Part model, mm, in its own coordinate system. Face numbers are marked on the shaded views. A direction names the side the tool comes from. Coordinates: 2 decimals unless noted, no trailing zeros. Loops run counter-clockwise (first coordinate to the right, second up) from the corner with the lowest first, then second, coordinate; pieces in that order, holes last. Notation, with made-up numbers: M 30,2.5 L 84,2.5 A9 cw 84,9.5 Z; hole C 8,42.5 d6. An arc over 180 degrees is marked long. Use a Markdown table: item, result. Add a question column.
1) Pin check, flat tips, straight feed: pin 1 Ø9.5 at (x, z) = (22, 0) entering from -Y; pin 2 Ø1 at (y, z) = (1, 0.5) entering from +X; pin 3 Ø6 at (x, z) = (5, -7) entering from +Y. Stop position of each tip, or through.
2) Band-saw the part on A-A (y = 1.25). List the corners of the cut face in (x, z), plus the area to 3 significant figures.
3) Band-saw the part on C-C (z = 2). List the corners of the cut face in (x, y), plus the area to 3 significant figures.
4) Pull direction X, two halves, no side cores. Call the marked faces 3, 4 and 5: released by +X, released by -X, zero draft, split by the parting line, or undercut.
5) Tool access for the marked faces 1 and 2: list every direction of +Z, -Z, +X, -X, +Y, -Y with a clear straight run to the whole face (end or side of a thin tool).
6) Wall check: probe 1 along X at (y, z) = (13.5, -7); probe 2 along Y at (x, z) = (29.5, 1.5); probe 3 along Y at (x, z) = (13.5, 10). Give the ranges that are in metal, low to high. Write a range as from..to.
7) Band-saw the part on B-B (x = 0). List the corners of the cut face in (y, z), plus the area to 3 significant figures.
from build123d import *

# Parameters (mm, degrees)
SKETCH_1_W          = 64
SKETCH_1_H          = 36
EXTRUDE_1_DEPTH     = 15.3
SKETCH_2_W          = 44
SKETCH_2_H          = 25
CUT_EXTRUDE_1_DEPTH = 2
SKETCH_3_W          = 16
SKETCH_3_H          = 6
CUT_EXTRUDE_2_DEPTH = 2


with BuildPart() as part:
    # 草图1 → 凸台-拉伸1 (new body)
    with BuildSketch(Plane(origin=(0, 0, 0), x_dir=(1, 0, 0), z_dir=(0, 1, 0))):
        Rectangle(SKETCH_1_W, SKETCH_1_H)
    extrude(amount=EXTRUDE_1_DEPTH)

    # 草图2 → 切除-拉伸1 (cut)
    with BuildSketch(Plane(origin=(0, 15.3, 0), x_dir=(1, 0, 0), z_dir=(0, 1, 0))):
        Rectangle(SKETCH_2_W, SKETCH_2_H)
    extrude(amount=-CUT_EXTRUDE_1_DEPTH, mode=Mode.SUBTRACT)

    # 草图3 → 切除-拉伸2 (cut)
    with BuildSketch(Plane.XZ):
        with Locations((24, -3)):
            Rectangle(SKETCH_3_W, SKETCH_3_H)
        with Locations((24, 3)):
            Rectangle(SKETCH_3_W, SKETCH_3_H)
    extrude(amount=-CUT_EXTRUDE_2_DEPTH, mode=Mode.SUBTRACT)


solid = part.part
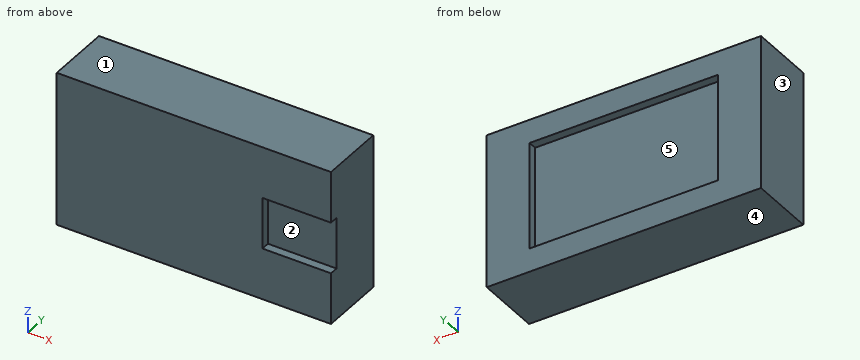
Entries:
| question | item | result |
|---|---|---|
| 1 | pin 1 | y = 2 |
| 1 | pin 2 | x = 16 |
| 1 | pin 3 | y = 13.3 |
| 2 | outline | M -32,-18 L 32,-18 L 32,-6 L 16,-6 L 16,6 L 32,6 L 32,18 L -32,18 Z |
| 2 | area | 2,110 mm2 |
| 3 | outline | M -32,0 L 16,0 L 16,2 L 32,2 L 32,15.3 L 22,15.3 L 22,13.3 L -22,13.3 L -22,15.3 L -32,15.3 Z |
| 3 | area | 859 mm2 |
| 4 | face 3 | released by -X |
| 4 | face 4 | zero draft |
| 4 | face 5 | undercut |
| 5 | face 1 | +Z, +X, -X, +Y, -Y |
| 5 | face 2 | +X, -Y |
| 6 | probe 1 | -32..-22, 22..32 |
| 6 | probe 2 | 2..15.3 |
| 6 | probe 3 | 0..13.3 |
| 7 | outline | M 0,-18 L 15.3,-18 L 15.3,-12.5 L 13.3,-12.5 L 13.3,12.5 L 15.3,12.5 L 15.3,18 L 0,18 Z |
| 7 | area | 501 mm2 |
